from build123d import *

# Parameters (mm, degrees)
SKETCH1_R           = 11
SKETCH1_R_2         = 2.5
SKETCH1_R_3         = 1.578075371
BOSS_EXTRUDE1_DEPTH = 2
SKETCH2_R           = 5
SKETCH2_R_2         = 2.5
BOSS_EXTRUDE2_DEPTH = 10
SKETCH3_R           = 1.5
CUT_EXTRUDE1_DEPTH  = 10.5


with BuildPart() as part:
    # Sketch1 → Boss-Extrude1 (new body)
    with BuildSketch(Plane.XY):
        Circle(SKETCH1_R)
        Circle(SKETCH1_R_2, mode=Mode.SUBTRACT)
        with Locations((-8.175, 0)):
            Circle(SKETCH1_R_3, mode=Mode.SUBTRACT)
        with Locations((0, 8.175)):
            Circle(SKETCH1_R_3, mode=Mode.SUBTRACT)
        with Locations((8.175, 0)):
            Circle(SKETCH1_R_3, mode=Mode.SUBTRACT)
        with Locations((0, -8.175)):
            Circle(SKETCH1_R_3, mode=Mode.SUBTRACT)
    extrude(amount=BOSS_EXTRUDE1_DEPTH)

    # Sketch2 → Boss-Extrude2 (add)
    with BuildSketch(Plane.XY.offset(2)):
        Circle(SKETCH2_R)
        Circle(SKETCH2_R_2, mode=Mode.SUBTRACT)
    extrude(amount=BOSS_EXTRUDE2_DEPTH)

    # Sketch3 → Cut-Extrude1 (cut, symmetric)
    with BuildSketch(Plane(origin=(0, 0, 0), x_dir=(1, 0, 0), z_dir=(0, 1, 0))):
        with Locations(Location((0, -7, 0), (0, 0, 270))):
            Circle(SKETCH3_R)
    extrude(amount=CUT_EXTRUDE1_DEPTH, both=True, mode=Mode.SUBTRACT)


solid = part.part
Geometry: final body of the model. Coordinates: model frame, mm. A direction names the side the tool comes from. Coordinates: 2 decimals unless noted, no trailing zeros. Order: outer loops, then holes, each group sorted by start corner. A loop starts at its lowest first (then second) coordinate and runs counter-clockwise, first axis right, second up.
1) Section A-A (y = 0). Return loops of the section in (x, z), then the cut area to 3 significant figures.
Result sheet:
outline: (-11, 0) - (-9.75, 0) - (-9.75, 2) - (-11, 2) - close; (-6.6, 0) - (-2.5, 0) - (-2.5, 12) - (-5, 12) - (-5, 2) - (-6.6, 2) - close; (2.5, 0) - (6.6, 0) - (6.6, 2) - (5, 2) - (5, 12) - (2.5, 12) - close; (9.75, 0) - (11, 0) - (11, 2) - (9.75, 2) - close
area: 71.4 mm2
2) First-contact query: P1, Ø2, axis at y = 8, z = 2.5, coming from the -X side; P2, Ø5, axis at x = 0, y = 8.175, coming from the +Z side; P3, Ø1.9, axis at x = 8.175, y = 0, coming from the -Z side; P4, Ø3, axis at x = -0.5, z = 9.5, coming from the +Y side. Flat tips, straight axial feed; report the tip coordinate or a pass-through.
Result sheet:
P1: stops at x = -8.37
P2: stops at z = 2
P3: passes through
P4: stops at y = 5
3) Section B-B (x = 0). Return loops of the section in (y, z).
Result sheet:
outline: (-11, 0) - (-9.75, 0) - (-9.75, 2) - (-11, 2) - close; (-6.6, 0) - (-2.5, 0) - (-2.5, 5.5) - (-5, 5.5) - (-5, 2) - (-6.6, 2) - close; (-5, 8.5) - (-2.5, 8.5) - (-2.5, 12) - (-5, 12) - close; (2.5, 0) - (6.6, 0) - (6.6, 2) - (5, 2) - (5, 5.5) - (2.5, 5.5) - close; (2.5, 8.5) - (5, 8.5) - (5, 12) - (2.5, 12) - close; (9.75, 0) - (11, 0) - (11, 2) - (9.75, 2) - close
4) Set-up query: faces 5 (the flat face through (0, 3, 0)), 6 (the cylindrical face through (2.307, -4.436, 6.93)). Return all of +Z, -Z, +X, -X, +Y, -Y with unobstructed straight access to the full face (end or side cutting, diameter ignored); none if empty.
Result sheet:
face 5: -Z, +X, -X, +Y, -Y
face 6: +Z
5) Section C-C (z = 7.25). Return loops of the section in (x, y).
Result sheet:
outline: (-1.48, -4.78) - (-1.48, -2.02) arc R2.5 cw to (-1.48, 2.02) - (-1.48, 4.78) arc R5 ccw to start; (1.48, -4.78) arc R5 ccw to (1.48, 4.78) - (1.48, 2.02) arc R2.5 cw to (1.48, -2.02) - close
6) Ray query, probe 1 along Y at (x, z) = (0, 1.25); probe 2 along Z at (x, y) = (0, 4.3); probe 3 along X at (y, z) = (-2, 10). Return the intervals inside material, ascending.
Result sheet:
probe 1: y = -11 to -9.75, -6.6 to -2.5, 2.5 to 6.6, 9.75 to 11
probe 2: z = 0 to 5.5, 8.5 to 12
probe 3: x = -4.58 to -1.5, 1.5 to 4.58
7) Section D-D (y = 8.75). Return loops of the section in (x, z), then the cut area to 3 significant figures.
Result sheet:
outline: (-6.67, 0) - (-1.47, 0) - (-1.47, 2) - (-6.67, 2) - close; (1.47, 0) - (6.67, 0) - (6.67, 2) - (1.47, 2) - close
area: 20.8 mm2
8) Draft query along Y for faces 1 (the cylindrical face through (6.6, 0.1, 1)), 2 (the cylindrical face through (-2.5, 0.1, 5.9)), 3 (the cylindrical face through (-2.38, -10.74, 0.99)), 4 (the cylindrical face through (-0.575, -3.482, 8.386)). Return one class per face: released by +Y, released by -Y, zero draft, split by the parting line, or undercut.
Result sheet:
face 1: undercut
face 2: undercut
face 3: split by the parting line
face 4: zero draft
